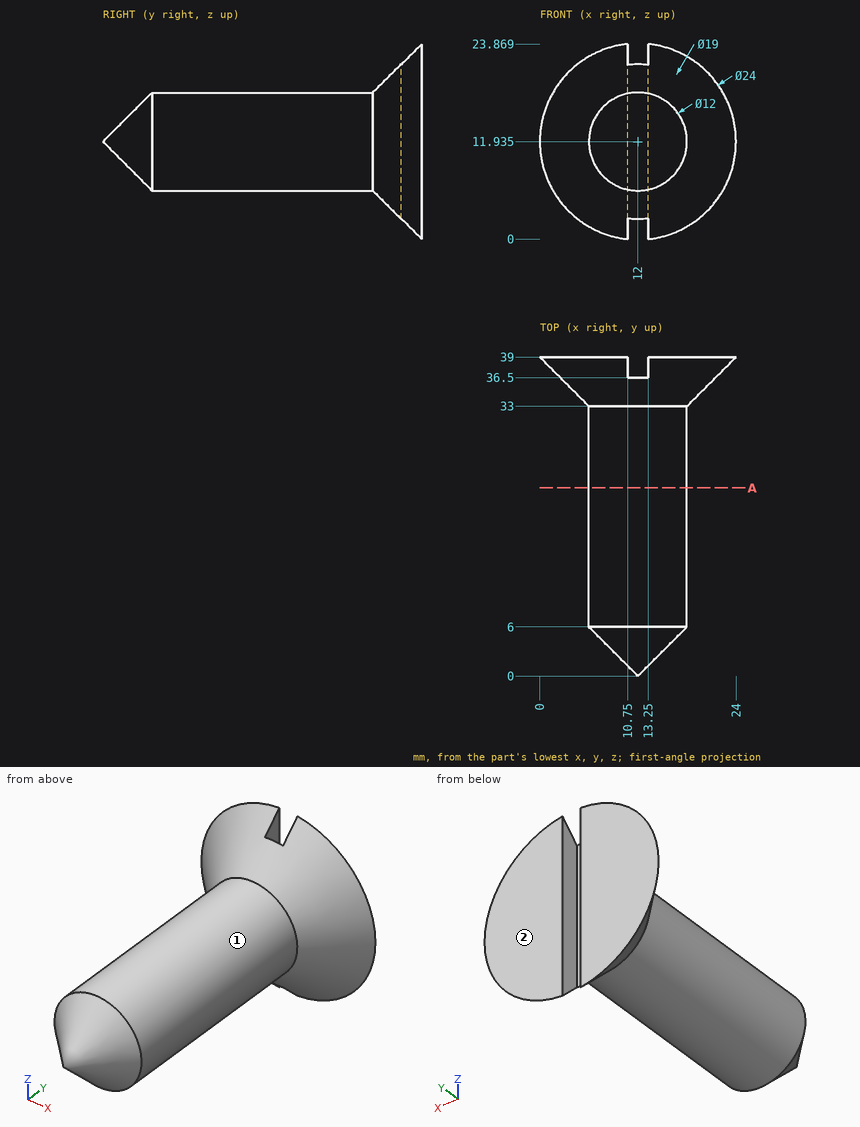
Design review of the part shown in the three views and the two pictorial views. Dimensions are in mm from the part's minimum x, y and z. A direction names the side the tool comes from. Coordinates: 2 decimals unless noted, no trailing zeros. Order: outer loops, then holes, each group sorted by start corner. A loop starts at its lowest first (then second) coordinate and runs counter-clockwise, first axis right, second up.
Item 1: For pin 1 Ø10 at (y, z) = (34, 6) entering from -X; pin 2 Ø3 at (y, z) = (37.5, 15) entering from +X (1 decimal); pin 3 Ø12 at (y, z) = (28, 11) entering from +X (1 decimal), all flat-tipped, find the tip position at first contact; note any pin that passes through.
Item 2: For the marked faces 1 and 2, list the 3-axis set-ups (+Z, -Z, +X, -X, +Y, -Y) from which the entire face can be reached by the end or side of a thin tool; tool diameter is ignored.
Item 3: Take a section at A-A, the plane y = 23. Write out the cut boundary in (x, z) (1 decimal).
Item 4: For line 1 (X direction, y = 31, z = 11.75); line 2 (Y direction, x = 4.25, z = 4.5); line 3 (Y direction, x = 7.25, z = 9.5), list the stretches that pass through material, from the lowest coordinate up.
The answers:
1. pin 1: stops at x = 1.09
1. pin 2: stops at x = 23.6
1. pin 3: stops at x = 19
2. face 1: -Y
2. face 2: +Z, -Z, +X, -X, +Y
3. outline: circle Ø12 at (12, 11.9)
4. line 1: x = 6 to 18
4. line 2: y = 37.74 to 39
4. line 3: y = 5.34 to 39
